Geometry: see drawing. Coordinates: mm, zero at the bounding-box minimum. A direction names the side the tool comes from. Coordinates: 2 decimals unless noted, no trailing zeros. Write each loop counter-clockwise with the first axis right and the second up, starting at its lowest first coordinate (ties: lowest second). Pieces come first, ordered by that corner, then holes. Notation, with made-up numbers: (-12, -15) - (-4, -15) arc R25 cw to (-4, 12) - close; hole circle Ø4 at (29, -18.5). An arc over 180 degrees is marked (long way). One line per question, with ' | ' between items. Start each with the question number.
1) Section query B-B on x = 17.25. Return loops of the section in (y, z).
2) Reachability of the marked faces 4, 5 and 6 from +Z, -Z, +X, -X, +Y, -Y: full face, straight path, thin tool, end or side. Return the list, or none.
3) Section query A-A on z = 17.25. Give the number of separate pieces and of enclosed holes in the cut face.
4) Line query: line 1 (Z direction, x = 17.25, y = 4.05); line 2 (Z direction, x = 17.25, y = 6.65); line 3 (Y direction, x = 9.5, z = 26). Output: solid intervals per line, ascending.
5) Draft query along X for the marked faces 1, 2 and 3. Return one class per face: released by +X, released by -X, zero draft, split by the parting line, or undercut.
6) First-contact query: P1, Ø5, axis at y = 3.5, z = 5.5, coming from the -X side; P2, Ø5, axis at x = 7, z = 12.5, coming from the -Y side; P3, Ø6, axis at x = 9.5, y = 4, coming from the -Z side; P4, Ø17, axis at x = 20.5, z = 9, coming from the -Y side. Flat tips, straight axial feed; report the tip coordinate or a pass-through.
7) Section query D-D on z = 10. Return loops of the section in (x, y).
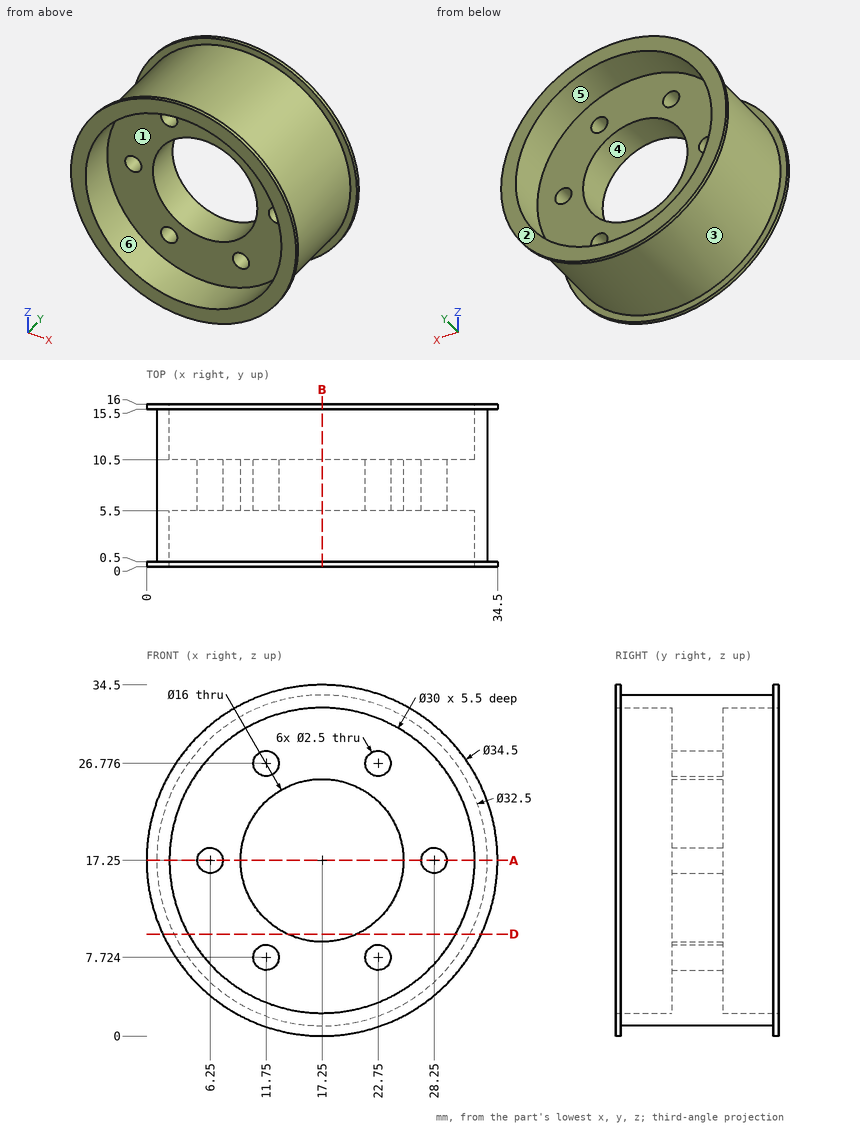
Answer key:
1) outline: (0, 0) - (0.5, 0) - (0.5, 1) - (15.5, 1) - (15.5, 0) - (16, 0) - (16, 2.25) - (10.5, 2.25) - (10.5, 9.25) - (5.5, 9.25) - (5.5, 2.25) - (0, 2.25) - close; (0, 32.25) - (5.5, 32.25) - (5.5, 25.25) - (10.5, 25.25) - (10.5, 32.25) - (16, 32.25) - (16, 34.5) - (15.5, 34.5) - (15.5, 33.5) - (0.5, 33.5) - (0.5, 34.5) - (0, 34.5) - close
2) face 4: +Y, -Y | face 5: +Y | face 6: -Y
3) separate pieces: 4 | enclosed holes: 0
4) line 1: 1 to 2.25, 32.25 to 33.5 | line 2: 1 to 9.25, 25.25 to 33.5 | line 3: 5.5 to 10.5
5) face 1: undercut | face 2: zero draft | face 3: split by the parting line
6) P1: x = 3.89 | P2: y = 5.5 | P3: z = 1.71 | P4: y = 0
7) outline: (1.6, 0) - (4.12, 0) - (4.12, 5.5) - (13.87, 5.5) - (13.87, 10.5) - (4.12, 10.5) - (4.12, 16) - (1.6, 16) - (1.6, 15.5) - (2.71, 15.5) - (2.71, 0.5) - (1.6, 0.5) - close; (20.63, 5.5) - (30.38, 5.5) - (30.38, 0) - (32.9, 0) - (32.9, 0.5) - (31.79, 0.5) - (31.79, 15.5) - (32.9, 15.5) - (32.9, 16) - (30.38, 16) - (30.38, 10.5) - (20.63, 10.5) - close
